Job drawing, mm, ordinate dimensions from the low corner. One solid piece. A direction names the side the tool comes from. Give positions to 0.01 mm unless a question says otherwise; leave off trailing zeros. Write each loop counter-clockwise with the first axis right and the second up, starting at its lowest first coordinate (ties: lowest second). Pieces come first, ordered by that corner, then holes. Notation, with made-up numbers: (89, 29.25) - (105, 29.25) arc R15 ccw to (105, 48.25) - close; hole circle Ø5 at (75, -13.75). An arc over 180 degrees is marked (long way). Use a Markdown table: item, result. Add a question column.
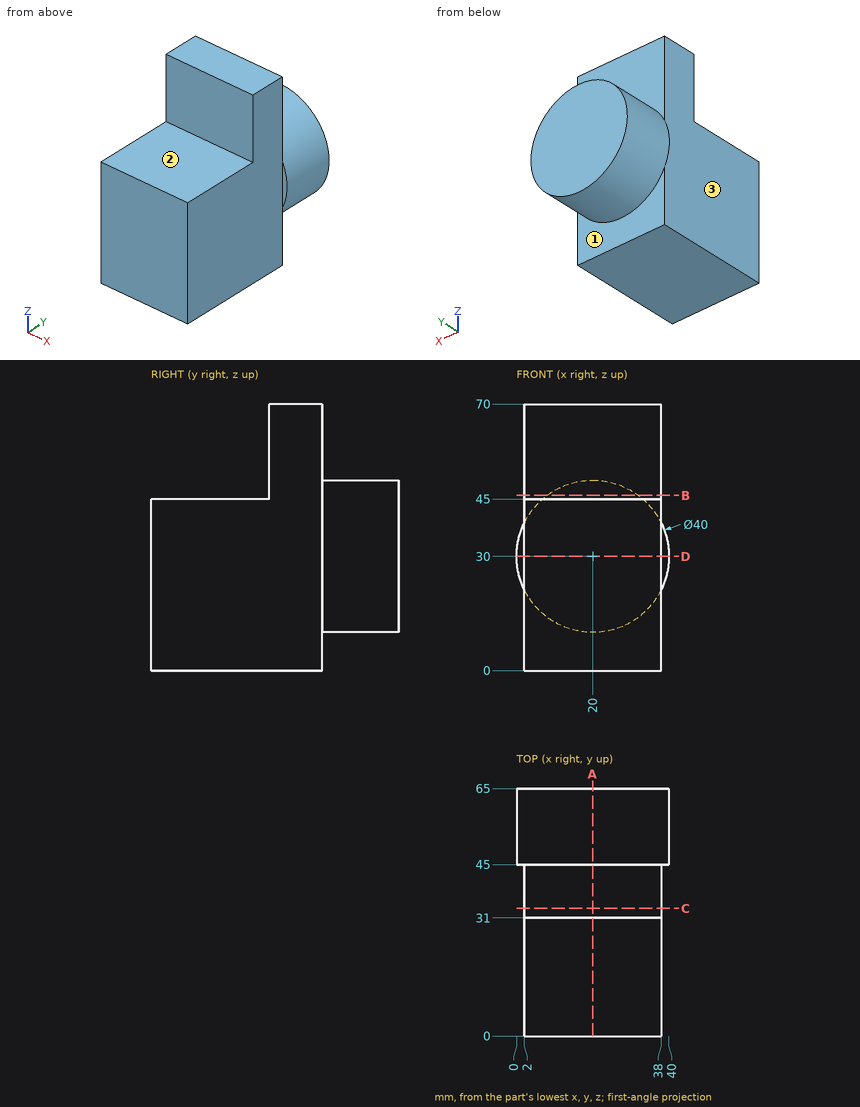
(1) Band-saw the part on D-D (z = 30). Write the cut outline in (x, y), then the cut area to 3 significant figures.
(2) Flat gauge pins, fed straight in: pin 1 (20 mm diameter, centred on x = 15, z = 59.5, fed in from -Y); pin 2 (10 mm diameter, centred on x = 12, y = 55, fed in from +Z); pin 3 (6 mm diameter, centred on y = 47, z = 8, fed in from -X). Where does each tip first touch, or does it go through?
(3) Band-saw the part on C-C (y = 33.5). Write the cut outline in (x, z).
(4) Probe probe 1 along Y at (x, z) = (34, 54.5); probe 2 along Z at (x, y) = (6, 20.5); probe 3 along X at (y, z) = (21, 8). List the from-to ranges inside material, lowest first. Write a range as [from, to].
(5) Band-saw the part on A-A (x = 20). Write the cut outline in (y, z).
(6) Which spindle directions (+Z, -Z, +X, -X, +Y, -Y) get a long thin tool onto all of the face, cutting with end or side? Do the marked faces 1, 2 and 3. Say none if no direction does.
(7) Band-saw the part on B-B (z = 46). Write the cut outline in (x, y).
Model answer:
| question | item | result |
|---|---|---|
| 1 | outline | (0, 45) - (2, 45) - (2, 0) - (38, 0) - (38, 45) - (40, 45) - (40, 65) - (0, 65) - close |
| 1 | area | 2,420 mm^2 |
| 2 | pin 1 | stops at y = 31 |
| 2 | pin 2 | stops at z = 49.77 |
| 2 | pin 3 | stops at x = 2 |
| 3 | outline | (2, 0) - (38, 0) - (38, 70) - (2, 70) - close |
| 4 | probe 1 | y = [31, 45] |
| 4 | probe 2 | z = [0, 45] |
| 4 | probe 3 | x = [2, 38] |
| 5 | outline | (0, 0) - (45, 0) - (45, 10) - (65, 10) - (65, 50) - (45, 50) - (45, 70) - (31, 70) - (31, 45) - (0, 45) - close |
| 6 | face 1 | -Z, +Y |
| 6 | face 2 | +Z, +X, -X, -Y |
| 6 | face 3 | +Z, -Z, -X, -Y |
| 7 | outline | (2, 31) - (38, 31) - (38, 45) - (32, 45) - (32, 65) - (8, 65) - (8, 45) - (2, 45) - close |
